from build123d import *

# Parameters (mm, degrees)
F0_R     = 56.3745675483
F1_DEPTH = 133.35
F2_R     = 25.4
F3_R     = 25.4
F4_T     = -2.54


# Not quite as in the source:
# - a shell that OpenCascade refuses in one call is made with other operations: the cavity is built on its own and cut out


with BuildPart() as f1:
    # F0 (on Top) → F1 (new body)
    with BuildSketch(Plane.XY):
        Circle(F0_R)
    extrude(amount=F1_DEPTH)

    # F2
    f2_edges = [f1.edges().sort_by_distance(p)[0] for p in [
        (-56.374568, 0, 133.35),
    ]]
    fillet(f2_edges, radius=F2_R)

    # F3
    f3_edges = [f1.edges().sort_by_distance(p)[0] for p in [
        (-56.374568, 0, 0),
    ]]
    fillet(f3_edges, radius=F3_R)

    # F4: a shell. OpenCascade refuses it in one call, so the cavity is built on its own and cut out:
    # the body offset inwards by the wall thickness, plus a prism from it out through each open face.
    f4_core = offset(f1.part, amount=F4_T, mode=Mode.PRIVATE)
    f4_exits = [f4_core.faces().sort_by_distance(p)[0] for p in [
        (0, 0, 2.54),
    ]]
    add(f4_core, mode=Mode.SUBTRACT)
    extrude(f4_exits, amount=-F4_T, mode=Mode.SUBTRACT)


solid = f1.part
Check sheet for the modelled part. Datum: model origin and axes. Units: mm. Round coordinates to 2 decimals unless told otherwise and drop trailing zeros. Loops run counter-clockwise (first coordinate to the right, second up) from the corner with the lowest first, then second, coordinate; pieces in that order, holes last. Notation, with made-up numbers: M -18.75,-9 L -7.75,-9 A34 ccw -7.75,27 Z; hole C 74,15.25 d7. An arc over 180 degrees is marked long. One line per item, written item: value.
(1) Sectioned sample at A-A, the plane y = 0. Record the cut outline in (x, z), then the cut area to 3 significant figures.
Computed values:
outline: M -56.37,25.4 A25.4 ccw -30.97,0 L -30.97,2.54 A22.86 cw -53.83,25.4 L -53.83,107.95 A22.86 cw -30.97,130.81 L 30.97,130.81 A22.86 cw 53.83,107.95 L 53.83,25.4 A22.86 cw 30.97,2.54 L 30.97,0 A25.4 ccw 56.37,25.4 L 56.37,107.95 A25.4 ccw 30.97,133.35 L -30.97,133.35 A25.4 ccw -56.37,107.95 Z
area: 962 mm^2
(2) Depth check by flat-ended pin: pin 1 Ø5 at (y, z) = (18, 89.5) entering from +X; pin 2 Ø6 at (x, z) = (30, 82) entering from -Y; pin 3 Ø1 at (y, z) = (37.5, 86) entering from -X. Enter the tip coordinate at first touch or a pass-through.
Computed values:
pin 1: stops at x = 54.2
pin 2: stops at y = -49.49
pin 3: stops at x = -42.53
(3) Sectioned sample at D-D, the plane z = 121. Record the cut outline in (x, y).
Computed values:
outline: C 0,0 d105.53; hole C 0,0 d99.49
(4) Thickness scan on line 1 (Y direction, x = 0, z = 51); line 2 (Z direction, x = -30, y = -9.5); line 3 (X direction, y = -1.5, z = 71.5). Record the ranges inside material, lowest first.
Computed values:
line 1: y = -56.37 to -53.83, 53.83 to 56.37
line 2: z = 0 to 2.55, 130.8 to 133.35
line 3: x = -56.35 to -53.81, 53.81 to 56.35
(5) Sectioned sample at C-C, the plane z = 34.5. Record the cut outline in (x, y), then the cut area to 3 significant figures.
Computed values:
outline: C 0,0 d112.75; hole C 0,0 d107.67
area: 879 mm^2
(6) Release check for a two-part mould opening along X. For faces 1 (the face through (28.613, -11.863, 1.288)), 2 (the face through (0, 0, 133.35)), 3 (the face through (-12.221, -55.034, 66.097)), 4 (the face through (51.35, 16.17, 66.1)) record: +X half, -X half, draft (parallel to the pull), parting line (faces both ways), or undercut.
Computed values:
face 1: undercut
face 2: draft
face 3: parting line
face 4: undercut
